Part model, mm, in its own coordinate system. A direction names the side the tool comes from. Round coordinates to 2 decimals unless told otherwise and drop trailing zeros. Order: outer loops, then holes, each group sorted by start corner. A loop starts at its lowest first (then second) coordinate and runs counter-clockwise, first axis right, second up. Notation, with made-up numbers: M 37,89 L 73,89 A25 cw 73,113 Z; hole C 42,16.5 d2. An arc over 180 degrees is marked long. Write each question's results on one line, items separated by ' | '. Start each with the question number.
1. Two-plate mould, pull along X, no slides. Class faces 5 (the face through (-17, -50.8, 15)), 6 (the face through (-15.202, -33.704, 15.028)), 7 (the face through (51.591, -25, 15)), 8 (the face through (6.61, -12.88, -17.94)): +X half, -X half, draft (parallel to the pull), parting line (faces both ways), or undercut.
2. Band-saw the part on C-C, the plane x = 12.5. List the corners of the cut face in (y, z), then the cut area to 3 significant figures.
3. Drop flat-ended pins along their axis: pin 1 Ø3 at (y, z) = (-28.5, -22) entering from -X; pin 2 Ø6 at (x, y) = (41.5, -22.5) entering from -Z; pin 3 Ø12.5 at (y, z) = (-13, -6) entering from -X; pin 4 Ø1.5 at (y, z) = (-9.5, -14.5) entering from +X. Give the stop position or say it passes through.
4. Band-saw the part on D-D, the plane y = -11. List the corners of the cut face in (x, z), then the cut area to 3 significant figures.
5. Probe L1, parallel to X at y = -38, z = 14; L2, parallel to Z at x = 36, y = -46.5; L3, parallel to Y at x = 4, z = -23.5. List the from-to ranges inside material, lowest first. Write a range as [from, to].
6. Band-saw the part on B-B, the plane y = -38.1. List the corners of the cut face in (x, z), then the cut area to 3 significant figures.
7. Which spindle directions (+Z, -Z, +X, -X, +Y, -Y) get a long thin tool onto all of the face, cutting with end or side? Do faces 1 (the face through (-6.412, -38, 15)), 2 (the face through (11, 0, 4)), 3 (the face through (-6.412, -13, -11)), 4 (the face through (30.313, -13, -11)). Say none if no direction does.
8. Band-saw the part on A-A, the plane z = 13. List the corners of the cut face in (x, y), then the cut area to 3 significant figures.
```python
from build123d import *

# Parameters (mm, degrees)
F0_W      = 79.5727856457
F0_H      = 52.4655748159
F1_DEPTH  = 25.4
F2_W      = 21.5691803023
F2_H      = 18.3629509993
F2_W_2    = 21.2777052075
F3_DEPTH  = 25.4
F4_W      = 21.5691803023
F4_H      = 34.1026238166
F4_W_2    = 21.2777052075
F5_DEPTH  = 25.4
F6_R      = 6.7292329965
F7_DEPTH  = 25.4
F8_R      = 4.9554758181
F9_DEPTH  = 25.4
F10_R     = 4.9823414423
F11_DEPTH = 25.4


with BuildPart() as f1:
    # F0 (on Front) → F1 (new body)
    with BuildSketch(Plane.XZ):
        with Locations((11.8047539145, -1.8945904449)):
            Rectangle(F0_W, F0_H)
    extrude(amount=F1_DEPTH)

    # F2 (on face) → F3 (join)
    with BuildSketch(Plane.XZ.offset(25.4)):
        with Locations((-17.1970487572, 15.1567214634)):
            Rectangle(F2_W, F2_H)
        with Locations((40.9522941336, 15.1567214634)):
            Rectangle(F2_W_2, F2_H)
    extrude(amount=F3_DEPTH)

    # F4 (on face) → F5 (cut)
    with BuildSketch(Plane.XZ.offset(25.4)):
        with Locations((-17.1970487572, -11.0760659445)):
            Rectangle(F4_W, F4_H)
        with Locations((40.9522941336, -11.0760659445)):
            Rectangle(F4_W_2, F4_H)
    extrude(amount=-F5_DEPTH, mode=Mode.SUBTRACT)

    # F6 (on face) → F7 (cut)
    with BuildSketch(Plane.XZ.offset(25.4)):
        with Locations((11.9504914619, -13.8450823724)):
            Circle(F6_R)
    extrude(amount=-F7_DEPTH, mode=Mode.SUBTRACT)

    # F8 (on face) → F9 (cut)
    with BuildSketch(Plane(origin=(0, 0, 5.9752459638), x_dir=(1, 0, 0), z_dir=(0, 0, -1))):
        with Locations((-17.4885243177, 38.1)):
            Circle(F8_R)
    extrude(amount=-F9_DEPTH, mode=Mode.SUBTRACT)

    # F10 (on face) → F11 (cut)
    with BuildSketch(Plane(origin=(0, 0, 5.9752459638), x_dir=(1, 0, 0), z_dir=(0, 0, -1))):
        with Locations((40.5150838196, 38.1)):
            Circle(F10_R)
    extrude(amount=-F11_DEPTH, mode=Mode.SUBTRACT)


solid = f1.part
```
Solution:
1) face 5: draft | face 6: undercut | face 7: +X half | face 8: undercut
2) outline: M -25.4,-28.13 L 0,-28.13 L 0,-20.55 L -25.4,-20.55 Z; M -25.4,-7.14 L 0,-7.14 L 0,24.34 L -25.4,24.34 Z | area: 992 mm^2
3) pin 1: through | pin 2: z = 5.98 | pin 3: x = -6.41 | pin 4: x = 30.31
4) outline: M -27.98,5.98 L -6.41,5.98 L -6.41,-28.13 L 30.31,-28.13 L 30.31,5.98 L 51.59,5.98 L 51.59,24.34 L -27.98,24.34 Z; hole C 11.95,-13.85 d13.46 | area: 2,570 mm^2
5) L1: [-27.98, -22.44], [-12.53, -6.41], [30.31, 35.53], [45.5, 51.59] | L2: [5.98, 24.34] | L3: [-25.4, 0]
6) outline: M -27.98,5.98 L -22.44,5.98 L -22.44,24.34 L -27.98,24.34 Z; M -12.53,5.98 L -6.41,5.98 L -6.41,24.34 L -12.53,24.34 Z; M 30.31,5.98 L 35.53,5.98 L 35.53,24.34 L 30.31,24.34 Z; M 45.5,5.98 L 51.59,5.98 L 51.59,24.34 L 45.5,24.34 Z | area: 422 mm^2
7) face 1: +Z, -Z, -Y | face 2: +Z, -Z, +X, -X, +Y | face 3: -Z, -X, +Y, -Y | face 4: -Z, +X, +Y, -Y
8) outline: M -27.98,-50.8 L -6.41,-50.8 L -6.41,-25.4 L 30.31,-25.4 L 30.31,-50.8 L 51.59,-50.8 L 51.59,0 L -27.98,0 Z; hole C -17.49,-38.1 d9.91; hole C 40.52,-38.1 d9.96 | area: 2,950 mm^2
